The listing builds one solid part. Answer for the finished solid, in the listing's coordinates (mm). A direction names the side the tool comes from. Round coordinates to 2 decimals unless told otherwise and drop trailing zeros. Loops run counter-clockwise (first coordinate to the right, second up) from the corner with the lowest first, then second, coordinate; pieces in that order, holes last. Notation, with made-up numbers: (-2.5, 42.25) - (15.5, 42.25) arc R29 cw to (15.5, 75.25) - close; hole circle Ø8 at (23.5, -24). An arc over 180 degrees is marked (long way). Write item = value, one per line. Start each with the question number.
1) A tool of negligible diameter and unlimited length cuts with its end or side. For faces 1 (the cylindrical face through (31.3, 8.2, 10.5)), 2 (the flat face through (24, -24.866, 14)), from which of +Z, -Z, +X, -X, +Y, -Y can it reach the whole face along a straight path? Write none if from no direction.
2) Section C-C, the plane x = 42 is taken. Determine the outline of the cut face in (y, z), and give its area (3 significant figures).
3) Section A-A, the plane y = 5.5 is taken. Determine the outline of the cut face in (x, z).
4) Given pin 1 Ø6 at (x, y) = (43.73, -19.47) entering from -Z; pin 2 Ø2.5 at (x, z) = (14, 9) entering from +Y; pin 3 Ø16 at (x, y) = (4.23, -4.87) entering from +Z, each flat-ended and moving along its own axis, determine where each tip first touches the part or whether it passes through.
5) Section D-D, the plane y = -7 is taken. Determine the outline of the cut face in (x, z).
6) Straight lines are drawn through the part: line 1 along X through (y, z) = (-9, 26.5); line 2 along X through (y, z) = (8.5, 19); line 3 along X through (y, z) = (10.5, 22.75). For each, find the intervals that lie inside material, in ascending order.
7) For a pull along X with two mould halves and no side action, classify faces 3 (the cylindrical face through (-7.6, 14.2, 14.2)), 4 (the cylindrical face through (17.035, 8.232, 17.749)), 5 (the flat face through (16, -5, 28)) as released by +X, released by -X, zero draft, split by the parting line, or undercut.
8) Section B-B, the plane z = 23 is taken. Give the number of separate pieces and of enclosed holes in the cut face, and give its area (3 significant figures).
Autodesk Inventor part; units mm, degrees
ref_plane "YZ Plane" through (0, 0, 0) normal (1, 0, 0) x (0, 1, 0)
ref_plane "XZ Plane" through (0, 0, 0) normal (0, 1, 0) x (-1, 0, 0)
ref_plane "XY Plane" through (0, 0, 0) normal (0, 0, 1) x (1, 0, 0)
sketch "Sketch1" plane through (0, 0, 0) normal (0, 0, 1) x (1, 0, 0)
  line L0 (-8.5249, 15.1341) -> (56.4751, 15.1341)
  line L1 (56.4751, 15.1341) -> (56.4751, -24.8659)
  line L2 (56.4751, -24.8659) -> (-8.5249, -24.8659)
  line L3 (-8.5249, -24.8659) -> (-8.5249, 15.1341)
  circle A0 centre (4.2251, -4.8659) radius 8.75
  line L4 (23.9751, 31.9095) -> (23.9751, -63.7078)
  circle A1 centre (43.7251, -4.8659) radius 8.75
  circle A2 centre (4.2251, 9.9285) radius 2.5
  circle A3 centre (4.2251, -19.471) radius 2.5
  circle A4 centre (43.7251, 9.9285) radius 2.5
  circle A5 centre (43.7251, -19.471) radius 2.5
  circle A6 centre (23.9751, -4.8659) radius 7.5
  point P0 (0, 0)
  dimension "d0" = 65
  dimension "d1" = 40
  dimension "d4" = 17.5
  dimension "d5" = 5
  dimension "d6" = 5
  dimension "d7" = 12.75
  dimension "d8" = 12.75
  dimension "d9" = 32.5
  dimension "d10" = 12.75
  dimension "d11" = 15
extrude "Extrusion1" add sketch "Sketch1" along normal blind 28 contours L0 L4 A6 L2 L3 | L0 L1 L2 L4 A6
fillet "Fillet1" radius 3.175 4 edges at (-8.5249, 15.1341, 14) (56.4751, 15.1341, 14) (56.4751, -24.8659, 14) (-8.5249, -24.8659, 14)
sketch "Sketch2" plane through (-5.3499, 15.1341, 0) normal (0, 1, 0) x (1, 0, 0)
  line L0 (58.65, 0) -> (58.65, -28)
  line L1 (0, 0) -> (58.65, 0)
  line L2 (0, -28) -> (0, 0)
  line L3 (0, -28) -> (58.65, -28)
  circle A0 centre (20, -9.5) radius 2.5
  circle A1 centre (38.65, -9) radius 2.5
  line L4 (-22.4443, -14) -> (82.6683, -14)
  circle A2 centre (20, -18.5) radius 2.5
  circle A3 centre (38.65, -19) radius 2.5
  point P0 (5.3499, 0)
  dimension "d15" = 5
  dimension "d16" = 5
  dimension "d19" = 20
  dimension "d21" = 20
  dimension "d22" = 4.5
  dimension "d23" = 5
  dimension "d24" = 14
  dimension "d25" = 28
extrude "Extrusion2" cut sketch "Sketch2" against normal blind 14 contours A0 | A1 | A2 | A3
thread "Thread1"
thread "Thread2"
thread "Thread3"
thread "Thread4"
equation "\"d7\" = d8"
equation "\"d10\" = d8"
equation "\"d21\" = d19"
equation "\"d23\" = d15"
equation "\"d24\" = 0.5 * d25"
properties part number "Mock Gearbox"
Geometry check:
q1.face_1 = +Y
q1.face_2 = +Z, -Z, +X, -X, -Y
q2.outline = (-24.87, 0) - (-21.28, 0) - (-21.28, 28) - (-24.87, 28) - close; (-17.66, 0) - (-13.44, 0) - (-13.44, 28) - (-17.66, 28) - close; (3.71, 0) - (8.12, 0) - (8.12, 28) - (3.71, 28) - close; (11.74, 0) - (15.13, 0) - (15.13, 28) - (11.74, 28) - close
q2.area = 437 mm2
q3.outline = (-8.52, 0) - (56.48, 0) - (56.48, 28) - (-8.52, 28) - close; hole circle Ø5 at (14.65, 9.5); hole circle Ø5 at (14.65, 18.5); hole circle Ø5 at (33.3, 9); hole circle Ø5 at (33.3, 19)
q4.pin_1 = 0
q4.pin_2 = 1.13
q4.pin_3 = through
q5.outline = (-8.52, 0) - (-4.26, 0) - (-4.26, 28) - (-8.52, 28) - close; (12.71, 0) - (16.79, 0) - (16.79, 28) - (12.71, 28) - close; (31.17, 0) - (35.24, 0) - (35.24, 28) - (31.17, 28) - close; (52.21, 0) - (56.48, 0) - (56.48, 28) - (52.21, 28) - close
q6.line_1 = -8.52 to -3.49, 11.94 to 17.72, 30.23 to 36.01, 51.44 to 56.48
q6.line_2 = -8.52 to 2.17, 6.28 to 12.2, 17.1 to 30.8, 35.8 to 41.67, 45.78 to 56.48
q6.line_3 = -8.52 to 1.79, 6.66 to 41.29, 46.16 to 56.48
q7.face_3 = released by -X
q7.face_4 = undercut
q7.face_5 = zero draft
q8.separate_pieces = 1
q8.enclosed_holes = 7
q8.area = 1,860 mm2
